Source: CAD feature listing. Evaluate the final solid. Frame: model axes, mm. Face numbers are marked on the shaded views. A direction names the side the tool comes from. Give positions to 0.01 mm unless a question says otherwise; leave off trailing zeros. Write each loop counter-clockwise with the first axis right and the second up, starting at its lowest first coordinate (ties: lowest second). Pieces come first, ordered by that corner, then holes. Notation, with made-up numbers: (-31, 50) -> (11, 50) arc R15 cw to (11, 65) -> close; hole circle Ø9 at (11, 45.5). An arc over 180 degrees is marked (long way). Use one line per item in the form item = value. Start each with the question number.
(1) Set-up query: the marked faces 1, 2, 3 and 4. Return all of +Z, -Z, +X, -X, +Y, -Y with unobstructed straight access to the full face (end or side cutting, diameter ignored); none if empty.
(2) Material intervals for line 1 along Z through (x, y) = (-7.5, 3); line 2 along X through (y, z) = (2.75, 0); line 3 along Z through (x, y) = (0, 1.75), sorted ascending. Write a range as from..to.
(3) Cut plane C-C, the plane z = -7.5. Output: boundary loops of the cut face in (x, y), and give its area (3 significant figures).
(4) Draft query along Z for the marked faces 5, 6, 7 and 8. Return one class per face: pulls with the +Z half, pulls with the -Z half, needs draft (parallel to the pull), parting line crosses it, or undercut.
(5) Cut plane D-D, the plane x = -7.5. Output: boundary loops of the cut face in (y, z), and give its area (3 significant figures).
(6) Cut plane A-A, the plane y = 3.75. Output: boundary loops of the cut face in (x, z).
(7) First-contact query: P1, Ø1, axis at x = -4.5, z = -1, coming from the +Y side; P2, Ø2.5, axis at y = 4, z = -7, coming from the +X side; P3, Ø1, axis at x = 0, y = 3, coming from the -Z side. Flat tips, straight axial feed; report the tip coordinate or a pass-through.
(8) Cut plane B-B, the plane x = 0. Output: boundary loops of the cut face in (y, z).
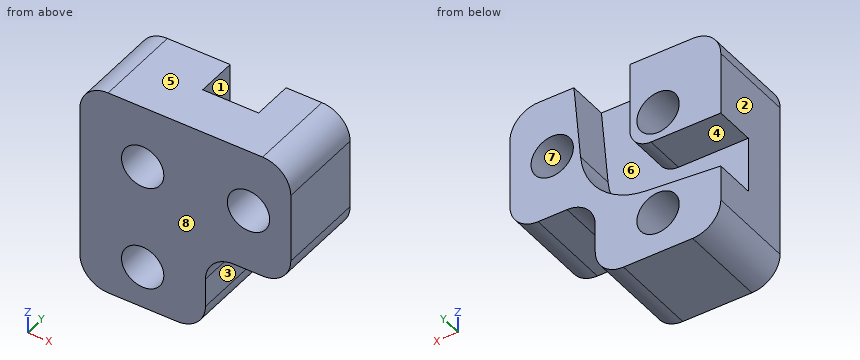
Autodesk Inventor part; units mm, degrees
ref_plane "YZ Plane" through (0, 0, 0) normal (1, 0, 0) x (0, 1, 0)
ref_plane "XZ Plane" through (0, 0, 0) normal (0, 1, 0) x (-1, 0, 0)
ref_plane "XY Plane" through (0, 0, 0) normal (0, 0, 1) x (1, 0, 0)
sketch "Sketch1" plane through (0, 0, 0) normal (0, 1, 0) x (-1, 0, 0)
  line L0 (0, 0) -> (7.5, 0) construction
  line L1 (7.5, 0) -> (7.5, -7.5) construction
  line L2 (0, 0) -> (-3, 0) construction
  line L3 (-3, -4.45) -> (-3, 4.45)
  line L4 (-3, 4.45) -> (11.95, 4.45)
  line L5 (11.95, 4.45) -> (11.95, -10.5)
  line L6 (11.95, -10.5) -> (3.05, -10.5)
  line L7 (3.05, -10.5) -> (3.05, -4.45)
  line L8 (3.05, -4.45) -> (-3, -4.45)
  line L9 (7.5, -7.5) -> (7.5, -10.5) construction
  dimension "d0" = 7.5
  dimension "d1" = 7.5
  dimension "d2" = 8.9
  dimension "d3" = 3
extrude "Extrusion1" add sketch "Sketch1" along normal blind 6.25
hole "Hole1" at (0, 0, 0) at (-7.5, 0, 0) at (-7.5, 0, -7.5) direction (0, 1, 0) diameter 3 end through all
sketch "Sketch2" plane through (0, 6.25, 0) normal (0, 1, 0) x (1, 0, 0)
  circle A0 centre (-7.5, 0) radius 1.5
  circle A1 centre (0, 0) radius 1.5 construction
  circle A2 centre (-7.5, 7.5) radius 1.5
  line L0 (3, -4.45) -> (3, 4.45) construction
  line L1 (3, 4.45) -> (-3.05, 4.45) construction
  line L2 (-3.05, 4.45) -> (-3.05, 10.5) construction
  line L3 (-3.05, 10.5) -> (-11.95, 10.5) construction
  line L4 (-11.95, 10.5) -> (-11.95, -4.45) construction
  line L5 (-11.95, -4.45) -> (3, -4.45) construction
  line L6 (-11.95, -4.45) -> (-11.95, 10.5)
  line L7 (-11.95, 2) -> (-7, 2)
  line L8 (-5.5, 2) -> (-5.5, 0.5) construction
  line L9 (-11.95, -4.45) -> (3, -4.45) construction
  line L10 (-3.05, 4.45) -> (3, 4.45) construction
  line L11 (-7.5, 0) -> (-7.5, 2) construction
  line L12 (-7.5, 0) -> (-5.5, 0) construction
  line L13 (-3.05, 4.45) -> (-3.05, 10.5) construction
  line L14 (-3.05, 10.5) -> (-3.05, 4.45) construction
  line L15 (-1.5378, -4.45) -> (-5.5, -4.45)
  line L16 (-11.95, 2) -> (-11.95, 5.9622)
  line L17 (-11.95, 10.5) -> (-11.95, -4.45)
  line L18 (-11.95, 5.9622) -> (-6.5633, 5.4909)
  line L19 (-1.5378, -4.45) -> (-2.0091, 0.9367)
  circle A3 centre (-7, 0.5) radius 1.5
  line L20 (-7, 2) -> (-5.5, 2) construction
  line L21 (-5.5, 0.5) -> (-5.5, -4.45)
  arc A4 (-2.0091, 0.9367) -> (-6.5633, 5.4909) centre (-7, 0.5) ccw
  dimension "d14" = 2
  dimension "d18" = 5
  dimension "d19" = 5
  dimension "d21" = 3
  dimension "d22" = 5.01
extrude "MontageEnForce" cut sketch "Sketch2" against normal blind 2.9 contours L7 L6 L18 A4 L19 L15 L21 A3
fillet "Fillet1" radius 2 6 edges at (-3.05, 3.125, -4.45) (-11.95, 3.125, 4.45) (-3.05, 3.125, -10.5) (-11.95, 3.125, -10.5) (3, 3.125, 4.45) (3, 3.125, -4.45)
ref_plane "Work Plane1" through (0, 4.8, 0) normal (0, 1, 0) x (1, 0, 0)
sketch "Sketch4" plane through (0, 6.25, 0) normal (0, 1, 0) x (1, 0, 0)
  circle A0 centre (-7.5, 0) radius 1.5
  circle A1 centre (-7.5, 7.5) radius 1.5
  circle A2 centre (0, 0) radius 1.5
ref_plane "Work Plane5" through (-7.5, 6.25, 0) normal (-1, 0, 0) x (0, 0, 1)
ref_plane "Work Plane6" through (0, 6.25, 0) normal (-1, 0, 0) x (0, 0, 1)
ref_plane "Work Plane7" through (-7.5, 6.25, 0) normal (0, 0, 1) x (1, 0, 0)
ref_plane "Work Plane8" through (-7.5, 6.25, -7.5) normal (0, 0, 1) x (1, 0, 0)
ref_plane "Work Plane2" through (-3.75, 6.25, 0) normal (-1, 0, 0) x (0, 0, 1)
ref_plane "Work Plane3" through (-7.5, 6.25, -3.75) normal (0, 0, 1) x (1, 0, 0)
equation "\"d0\" = side_2_corner"
equation "\"d1\" = side_2_corner"
equation "\"d2\" = width"
equation "\"d3\" = hole_2_border"
equation "\"d4\" = fix_thickness"
equation "\"d14\" = wire_2_corner"
equation "\"d18\" = angle_tol"
equation "\"d19\" = angle_tol"
equation "\"d21\" = 2 * wire_corner_fillet"
equation "\"d22\" = wire_corner_margin + wire_diameter + wire_corner_fillet"
equation "\"fix_thickness\" = 6.25"
equation "\"wire_diameter\" = 3"
equation "\"back_fix_width\" = 1"
equation "\"side_2_corner\" = piano_wire_holes_spacing"
equation "\"wire_2_corner\" = 2"
equation "\"angle_tol\" = 5deg"
equation "\"wire_corner_margin\" = 0.51"
equation "\"wire_corner_fillet\" = 1.5"
equation "\"hole_2_border\" = 3"
properties part number "piano_wire_back_fixation"
Geometry says:
q1.face_1 = +Z, +Y
q1.face_2 = +Z, -Z, -X, +Y, -Y
q1.face_3 = -Z, +X, +Y, -Y
q1.face_4 = -X, +Y
q2.line_1 = -10.5..-9, -6..-1.5, 1.5..4.45
q2.line_2 = -11.95..-9, -6..-1.5, 1.5..3
q2.line_3 = -4.45..-1.5, 1.5..4.45
q3.outline = (-11.95, 0) -> (-9, 0) -> (-9, 6.25) -> (-11.95, 6.25) -> close; (-6, 0) -> (-3.05, 0) -> (-3.05, 6.25) -> (-6, 6.25) -> close
q3.area = 36.9 mm^2
q4.face_5 = pulls with the +Z half
q4.face_6 = undercut
q4.face_7 = undercut
q4.face_8 = needs draft
q5.outline = (0, -10.5) -> (6.25, -10.5) -> (6.25, -9) -> (0, -9) -> close; (0, -6) -> (6.25, -6) -> (6.25, -5.57) -> (3.35, -5.57) -> (3.35, -2) -> (6.25, -2) -> (6.25, -1.5) -> (0, -1.5) -> close; (0, 1.5) -> (6.25, 1.5) -> (6.25, 4.45) -> (0, 4.45) -> close
q5.area = 45.6 mm^2
q6.outline = (-11.95, -8.5) arc R2 ccw to (-9.95, -10.5) -> (-5.05, -10.5) arc R2 ccw to (-3.05, -8.5) -> (-3.05, -6.45) arc R2 cw to (-1.05, -4.45) -> (1, -4.45) arc R2 ccw to (3, -2.45) -> (3, 2.45) arc R2 ccw to (1, 4.45) -> (-1.54, 4.45) -> (-2.01, -0.94) arc R5.01 cw to (-6.56, -5.49) -> (-11.95, -5.96) -> close; (-11.95, -2) -> (-7, -2) arc R1.5 ccw to (-5.5, -0.5) -> (-5.5, 4.45) -> (-9.95, 4.45) arc R2 ccw to (-11.95, 2.45) -> close; hole circle Ø3 at (-7.5, -7.5); hole circle Ø3 at (-7.5, 0); hole circle Ø3 at (0, 0)
q7.P1 = 3.35
q7.P2 = -2.92
q7.P3 = -4.45
q8.outline = (0, -4.45) -> (6.25, -4.45) -> (6.25, -1.5) -> (0, -1.5) -> close; (0, 1.5) -> (6.25, 1.5) -> (6.25, 4.45) -> (0, 4.45) -> close
